Design review of the part built by this model. Coordinates are the model's own, in mm. A direction names the side the tool comes from. Give positions to 0.01 mm unless a question says otherwise; leave off trailing zeros. Order: outer loops, then holes, each group sorted by start corner. A loop starts at its lowest first (then second) coordinate and runs counter-clockwise, first axis right, second up. Notation, with made-up numbers: (76.5, 75.25) -> (132.5, 75.25) arc R16 cw to (132.5, 82.25) -> close; hole circle Ø7 at (61, 88). An arc over 180 degrees is marked (long way). One line per item, written item: value.
from build123d import *

# Parameters (mm, degrees)
PAD017_DEPTH    = 10
SKETCH043_R     = 2.5
HOLE004_DEPTH   = 74.4118637621
POCKET018_DEPTH = 21.6598644736
SKETCH071_R     = 3
PAD030_DEPTH    = 8
SKETCH072_R     = 2.5
POCKET034_DEPTH = 8
SKETCH073_W     = 3
SKETCH073_H     = 14
PAD031_DEPTH    = 4
SKETCH074_W     = 3
SKETCH074_H     = 14
PAD032_DEPTH    = 4


with BuildPart() as part:
    # Sketch041 → Pad017 (new body)
    with BuildSketch(Plane.YZ):
        Polygon((-9.2823155717, -17.4697729947), (-9.2823155717, -22.4697729947), (0, -22.4697729947), (0, -32.4697729947), (-9.2823155717, -32.4697729947), (-9.2823155717, -37.4697729947), (0.718202267, -37.4697729947), (16.14, -32.4697729947), (61.14, -39.1286374683), (61.14, -15.9992606277), (16.14, -22.4697729947), (0.718202267, -17.4697729947), align=None)
    extrude(amount=PAD017_DEPTH)

    # Sketch043 → Hole004 (cut, through all)
    with BuildSketch(Plane.ZX.offset(65.1285481904)):
        with Locations((-27.248053, 5.238883)):
            Circle(SKETCH043_R)
    extrude(amount=-HOLE004_DEPTH, mode=Mode.SUBTRACT)

    # Sketch044 (on Face2 of Hole004) → Pocket018 (cut, through all)
    with BuildSketch(Plane(origin=(0, 0, -17.4697729947), x_dir=(0, -1, 0), z_dir=(0, 0, 1))):
        with BuildLine():
            ThreePointArc((2.4, -6.9475921725), (5, -9.5475921725), (7.6, -6.9475921725))
            Line((7.6, -6.9475921725), (7.6, 6))
            ThreePointArc((7.6, 6), (5.0000000001, 8.6), (2.4, 6.0000000001))
            Line((2.4, -6.9475921725), (2.4, 6.0000000001))
        make_face()
    extrude(amount=-POCKET018_DEPTH, mode=Mode.SUBTRACT)

    # Sketch071 (on Face17 of Pocket018) → Pad030 (join)
    with BuildSketch(Plane.ZX.offset(61.14)):
        with Locations((-27.24572, 5.247846)):
            Circle(SKETCH071_R)
    extrude(amount=PAD030_DEPTH)

    # Sketch072 (on Face26 of Pad030) → Pocket034 (cut)
    with BuildSketch(Plane.ZX.offset(69.14)):
        with Locations((-27.257469, 5.237027)):
            Circle(SKETCH072_R)
    extrude(amount=-POCKET034_DEPTH, mode=Mode.SUBTRACT)

    # Sketch073 (on Face6 of Pocket034) → Pad031 (join)
    with BuildSketch(Plane(origin=(0, 0, 0), x_dir=(0, 1, 0), z_dir=(-1, 0, 0))):
        with Locations((59.6559768039, 27.292839)):
            Rectangle(SKETCH073_W, SKETCH073_H)
    extrude(amount=PAD031_DEPTH)

    # Sketch074 (on Face5 of Pad031) → Pad032 (join)
    with BuildSketch(Plane.YZ.offset(10)):
        with Locations((59.6497417125, -27.3033236781)):
            Rectangle(SKETCH074_W, SKETCH074_H)
    extrude(amount=PAD032_DEPTH)


with BuildPart() as part_1:
    # Body007 placement: moved
    add(part.part.moved(Location((0, -4, -37))))


solid = part_1.part
Item 1: Clearance check with flat-ended pins moving along their axes: P1, Ø1.5, axis at y = 16.5, z = -72.5, coming from the +X side; P2, Ø0.9, axis at x = -1, y = 55.5, coming from the +Z side; P3, Ø1.9, axis at y = -12.5, z = -57, coming from the -X side; P4, Ø4, axis at x = 6.5, y = 22.5, coming from the -Z side. State where each tip first meets the part, or that it passes through.
Returned:
P1: through
P2: z = -57.29
P3: x = 0
P4: z = -71.3
Item 2: Draft analysis for pull direction Z (two halves, no side actions). For faces 1 (the flat face through (12, 54.15, -64)), 2 (the flat face through (7.2, -6.5, -69.47)), 3 (the flat face through (12, 56, -71.303)), 4 (the flat face through (3, -4, -66)), state which applies: pulls with the +Z half, pulls with the -Z half, needs draft (parallel to the pull), parting line crosses it, or undercut.
Returned:
face 1: needs draft
face 2: undercut
face 3: pulls with the -Z half
face 4: undercut
Item 3: Add section B-B on y = 23.5. Give the boundary of the cut face in (x, z).
Returned:
outline: (0, -71.15) -> (10, -71.15) -> (10, -57.84) -> (0, -57.84) -> close; hole circle Ø5 at (5.24, -64.25)
Item 4: Add section D-D on y = 47. Give the boundary of the cut face in (x, z).
Returned:
outline: (0, -74.63) -> (10, -74.63) -> (10, -54.46) -> (0, -54.46) -> close; hole circle Ø5 at (5.24, -64.25)
Item 5: Add section C-C on x = -2. Give the boundary of the cut face in (y, z).
Returned:
outline: (54.16, -71.29) -> (57.16, -71.29) -> (57.16, -57.29) -> (54.16, -57.29) -> close
Item 6: Machinability: for faces 5 (the flat face through (4.93, 34.325, -72.753)), 6 (the flat face through (-2, 56, -71.293)), 7 (the flat face through (3, -6.4, -72)), which of the approach directions +Z, -Z, +X, -X, +Y, -Y give a long, thin tool a straight path to every point of the face, cutting with its end or side? Answer none if there is none.
Returned:
face 5: -Z, +X, -X
face 6: -Z, -X, +Y, -Y
face 7: +Z, -Z, -X
Item 7: To check wall thickness, follow line 1 along X through (y, z) = (60, -64.25); line 2 along X through (y, z) = (32.5, -60.5); line 3 along Z through (x, y) = (6.25, 5). State the ranges of each line that lie inside material, in increasing order. Write a range as from..to.
Returned:
line 1: 2.25..2.74, 7.74..8.25
line 2: 0..10
line 3: -71.78..-66.53, -61.96..-57.15
Item 8: Add section A-A on y = -9. Give the boundary of the cut face in (x, z).
Returned:
outline: (8.6, -74.47) -> (10, -74.47) -> (10, -69.47) -> (8.6, -69.47) -> close; (8.6, -59.47) -> (10, -59.47) -> (10, -54.47) -> (8.6, -54.47) -> close
